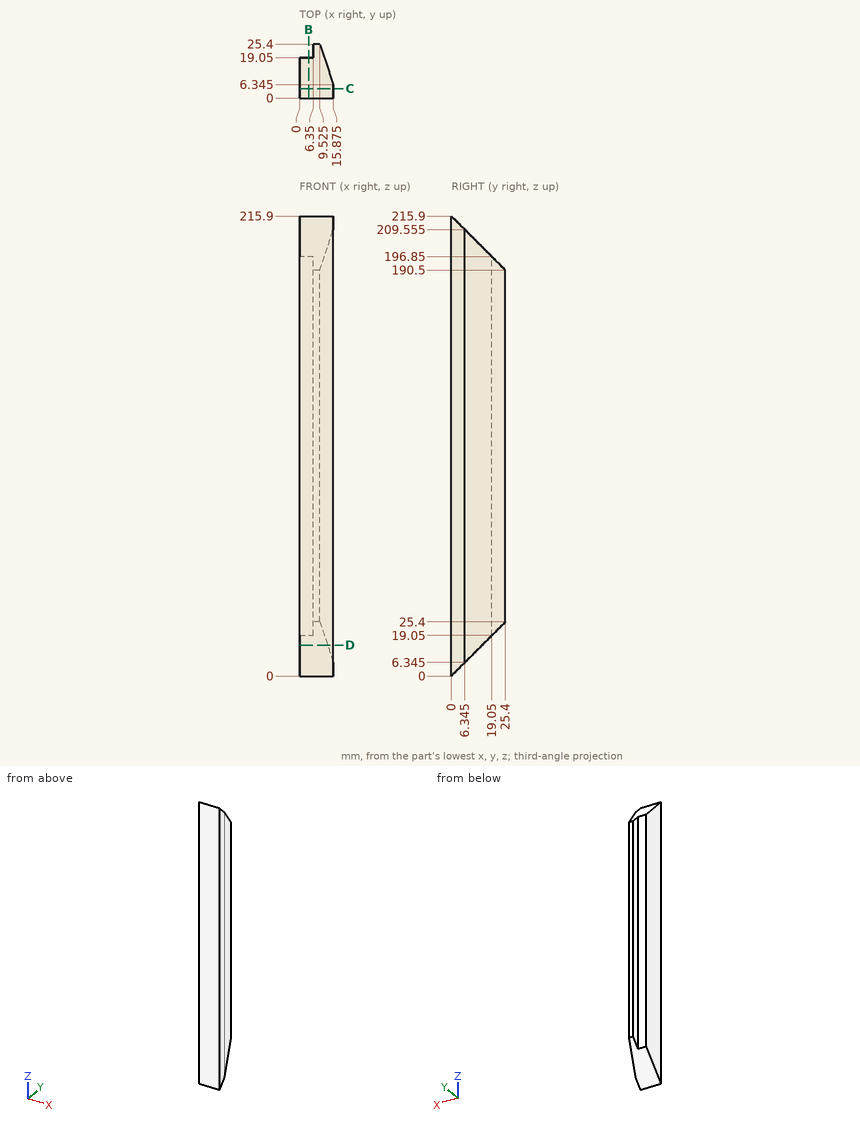
Part print with two shaded views. Sizes in mm from the minimum x, y, z corner. Round coordinates to 2 decimals unless told otherwise and drop trailing zeros. Order: outer loops, then holes, each group sorted by start corner. A loop starts at its lowest first (then second) coordinate and runs counter-clockwise, first axis right, second up. Notation, with made-up numbers: (17.5, -25) - (40.5, -25) arc R6 cw to (40.5, -17) - close; hole circle Ø5 at (-22, 49.25). An arc over 180 degrees is marked (long way). Answer in a Markdown table with one row per item. Add a question column.
(1) Band-saw the part on B-B on x = 4.25. List the corners of the cut face in (y, z).
(2) Probe L1, parallel to Y at x = 5, z = 36.5; L2, parallel to Z at x = 2.75, y = 9; L3, parallel to Z at x = 13.5, y = 3.25. List the from-to ranges inside material, lowest first. Write a range as [from, to].
(3) Band-saw the part on D-D on z = 14.5. List the corners of the cut face in (x, y) (1 decimal).
(4) Drop flat-ended pins along their axis: pin 1 Ø6 at (y, z) = (22.5, 131) entering from -X; pin 2 Ø8 at (x, y) = (11.5, 16) entering from +Z; pin 3 Ø1 at (x, y) = (8, 14.5) entering from +Z. Give the stop position or say it passes through.
(5) Band-saw the part on C-C on y = 4.5. List the corners of the cut face in (x, z) (1 decimal).
Data:
| question | item | result |
|---|---|---|
| 1 | outline | (0, 0) - (19.05, 19.05) - (19.05, 196.85) - (0, 215.9) - close |
| 2 | L1 | y = [0, 19.05] |
| 2 | L2 | z = [9, 206.9] |
| 2 | L3 | z = [3.25, 212.65] |
| 3 | outline | (0, 0) - (15.9, 0) - (15.9, 6.3) - (13.2, 14.5) - (0, 14.5) - close |
| 4 | pin 1 | stops at x = 6.35 |
| 4 | pin 2 | stops at z = 203.9 |
| 4 | pin 3 | stops at z = 201.9 |
| 5 | outline | (0, 4.5) - (15.9, 4.5) - (15.9, 211.4) - (0, 211.4) - close |
